Part print with two shaded views. Sizes in mm from the minimum x, y, z corner. A direction names the side the tool comes from. Round coordinates to 2 decimals unless told otherwise and drop trailing zeros. Loops run counter-clockwise (first coordinate to the right, second up) from the corner with the lowest first, then second, coordinate; pieces in that order, holes last.
(1) Cut at D-D on x = 6.5. List the corners of the cut face in (y, z), then the cut area to 3 significant figures.
(2) Cut at B-B on z = 8. List the corners of the cut face in (x, y).
(3) Tool access for the marked faces 5 and 6: list every direction of +Z, -Z, +X, -X, +Y, -Y with a clear straight run to the whole face (end or side of a thin tool).
(4) Probe probe 1 along Z at (x, y) = (35, 0.25); probe 2 along X at (y, z) = (0.45, 5); probe 3 along X at (y, z) = (4.25, 3). List the from-to ranges inside material, lowest first.
(5) Cut at A-A on x = 15. List the corners of the cut face in (y, z), then the cut area to 3 significant figures.
(6) Cut at C-C on y = 6.5. List the corners of the cut face in (x, z).
(7) Mould opens along X. For the marked faces 1, 2, 3 and 4 say: +X half, -X half, draft (parallel to the pull), parting line (faces both ways), or undercut.
(8) Flat gauge pin, fed straight in: pin 1 (5 mm diameter, centred on x = 27.5, z = 6, fed in from +Y). Where does the tip first touch, or does it go through?
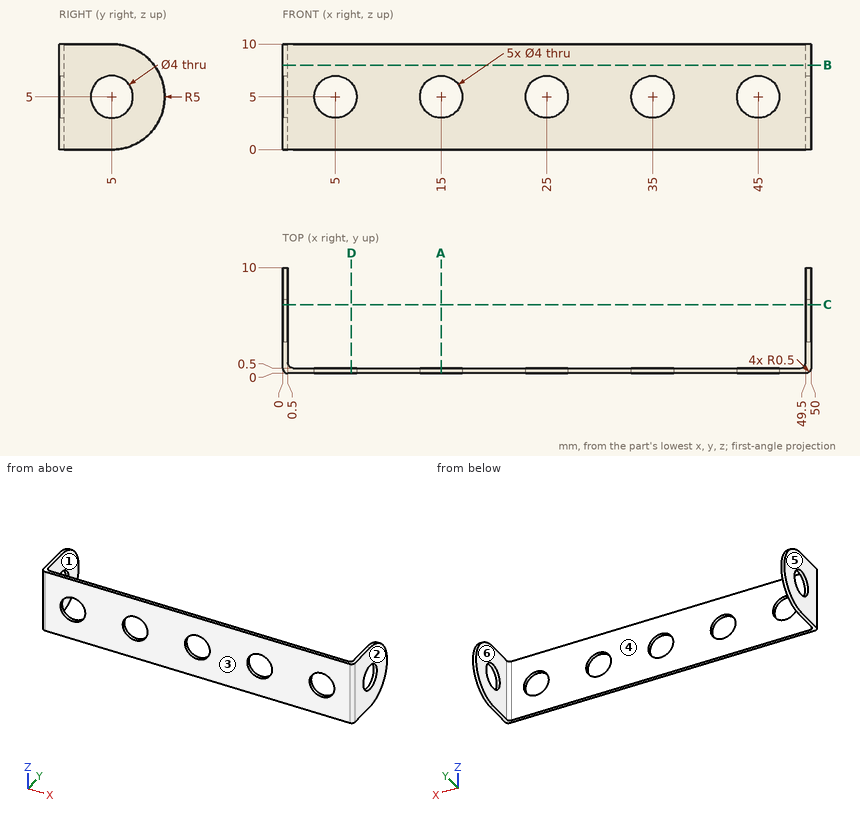
Final values:
1. outline: (0, 0) - (0.5, 0) - (0.5, 3.68) - (0, 3.68) - close; (0, 6.32) - (0.5, 6.32) - (0.5, 10) - (0, 10) - close
1. area: 3.68 mm2
2. outline: (0, 0.5) arc R0.5 ccw to (0.5, 0) - (49.5, 0) arc R0.5 ccw to (50, 0.5) - (50, 9) - (49.5, 9) - (49.5, 1) arc R0.5 cw to (49, 0.5) - (1, 0.5) arc R0.5 cw to (0.5, 1) - (0.5, 9) - (0, 9) - close
3. face 5: +Z, -Z, -X, +Y, -Y
3. face 6: +Z, -Z, +Y
4. probe 1: z = 0 to 3, 7 to 10
4. probe 2: x = 0 to 3, 7 to 13, 17 to 23, 27 to 33, 37 to 43, 47 to 50
4. probe 3: x = 0 to 0.5, 49.5 to 50
5. outline: (0, 0) - (0.5, 0) - (0.5, 3) - (0, 3) - close; (0, 7) - (0.5, 7) - (0.5, 10) - (0, 10) - close
5. area: 3.00 mm2
6. outline: (0, 0.23) - (0.5, 0.23) - (0.5, 3.68) - (0, 3.68) - close; (0, 6.32) - (0.5, 6.32) - (0.5, 9.77) - (0, 9.77) - close; (49.5, 0.23) - (50, 0.23) - (50, 3.68) - (49.5, 3.68) - close; (49.5, 6.32) - (50, 6.32) - (50, 9.77) - (49.5, 9.77) - close
7. face 1: undercut
7. face 2: +X half
7. face 3: draft
7. face 4: undercut
8. pin 1: stops at y = 0.5
